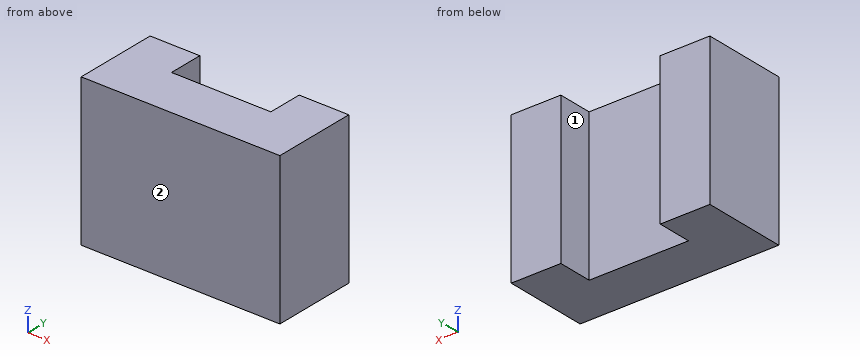
```python
from build123d import *

# Parameters (mm, degrees)
SKETCH1_W           = 20
SKETCH1_H           = 15
BOSS_EXTRUDE1_DEPTH = 5
SKETCH3_W           = 5
SKETCH3_H           = 3.480811901
BOSS_EXTRUDE2_DEPTH = 15


with BuildPart() as part:
    # Sketch1 → Boss-Extrude1 (new body)
    with BuildSketch(Plane(origin=(0, 0, 0), x_dir=(1, 0, 0), z_dir=(0, 1, 0))):
        with Locations((10, 7.5)):
            Rectangle(SKETCH1_W, SKETCH1_H)
    extrude(amount=BOSS_EXTRUDE1_DEPTH)

    # Sketch3 → Boss-Extrude2 (add)
    with BuildSketch(Plane.XY):
        with Locations((2.5, 6.740405951)):
            Rectangle(SKETCH3_W, SKETCH3_H)
        with Locations((17.5, 6.740405951)):
            Rectangle(SKETCH3_W, SKETCH3_H)
    extrude(amount=-BOSS_EXTRUDE2_DEPTH)


solid = part.part
```
Here's how the part is built. I have some questions about the finished solid (model axes, mm). Face numbers are marked on the shaded views. A direction names the side the tool comes from. Round coordinates to 2 decimals unless told otherwise and drop trailing zeros. Order: outer loops, then holes, each group sorted by start corner. A loop starts at its lowest first (then second) coordinate and runs counter-clockwise, first axis right, second up. Notation, with made-up numbers: M -9,81.25 L -4,81.25 A14 cw -4,107.25 Z; hole C 44,47 d10. An arc over 180 degrees is marked long. Answer in a Markdown table with one row per item.
Item 1: If I drill on L1, parallel to X at y = 7.5, z = -7; L2, parallel to Y at x = 10.5, z = -3.75, over which ranges is the centre line in solid material (lowest first)? Write a range as from..to.
A:
| item | result |
|---|---|
| L1 | x = 0..5, 15..20 |
| L2 | y = 0..5 |
Item 2: Imagine slicing it at B-B, the plane x = 10.5. Write out the boundary of the cut face in (y, z), and give its area (3 significant figures).
A:
| item | result |
|---|---|
| outline | M 0,-15 L 5,-15 L 5,0 L 0,0 Z |
| area | 75.0 mm2 |
Item 3: I'm going to push a flat-ended pin straight in: pin 1 (5 mm diameter, centred on x = 11.5, z = -7, fed in from +Y). Where does the tip first touch, or does it pass through?
A:
| item | result |
|---|---|
| pin 1 | stops at y = 5 |
Item 4: For the marked faces 1 and 2, which set-ups out of +Z, -Z, +X, -X, +Y, -Y let a thin tool reach every point of the face, with its end or its side?
A:
| item | result |
|---|---|
| face 1 | +Z, -Z, +Y |
| face 2 | +Z, -Z, +X, -X, -Y |
Item 5: Imagine slicing it at A-A, the plane z = -6.5. Write out the boundary of the cut face in (x, y), and give its area (3 significant figures).
A:
| item | result |
|---|---|
| outline | M 0,0 L 20,0 L 20,8.48 L 15,8.48 L 15,5 L 5,5 L 5,8.48 L 0,8.48 Z |
| area | 135 mm2 |
